Input: dimensioned drawing with shaded views. Units: mm. Origin: part minimum x, y, z. A direction names the side the tool comes from. Round coordinates to 2 decimals unless told otherwise and drop trailing zeros. Write each loop counter-clockwise with the first axis right and the second up, starting at its lowest first coordinate (ties: lowest second). Pieces come first, ordered by that corner, then holes. Notation, with made-up numbers: M -13.75,87.25 L 13.25,87.25 A33 ccw 13.25,115.25 Z; hole C 59,36 d9. An arc over 180 degrees is marked long. Answer as CSV lines item,"result". Start each with the question number.
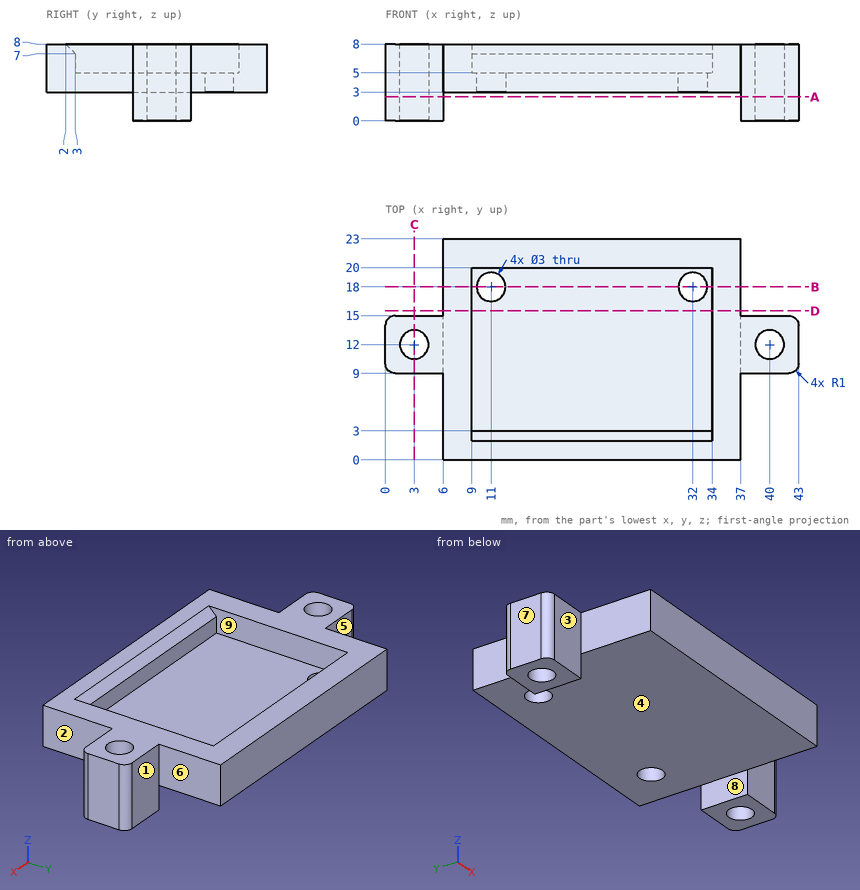
Item 1: Cut plane B-B, the plane y = 18. Return loops of the section in (x, z).
Item 2: Cut plane A-A, the plane z = 2.5. Return loops of the section in (x, y).
Item 3: Pin query (flat end, axial travel): pin 1 Ø1 at (x, y) = (24.5, 17) entering from +Z; pin 2 Ø7 at (x, y) = (15.5, 9.5) entering from -Z; pin 3 Ø2.5 at (x, z) = (38.5, 5) entering from -Y; pin 4 Ø2.5 at (x, y) = (11, 18) entering from -Z. Return the tip coordinate at first contact, or that it passes through.
Item 4: Line query: line 1 (Y direction, x = 3, z = 4.25); line 2 (Y direction, x = 17, z = 5.75); line 3 (X direction, y = 16.75, z = 3.25). Output: solid intervals per line, ascending. Write a range as [from, to].
Item 5: Cut plane D-D, the plane y = 15.5. Return loops of the section in (x, z).
Item 6: Access query for the marked faces 1, 2, 3, 4 and 5. Directions: +Z, -Z, +X, -X, +Y, -Y. A direction counts if a zero-diameter tool reaches every point of the face in a straight line with its end or side. Return the directions, or none.
Item 7: Draft query along X for the marked faces 6, 7, 8 and 9. Return one class per face: +X half, -X half, draft (parallel to the pull), parting line (faces both ways), or undercut.
Item 8: Cut plane C-C, the plane x = 3. Return loops of the section in (y, z), plus the area to 3 significant figures.
Results list:
1,outline,"M 6,3 L 9.5,3 L 9.5,5 L 9,5 L 9,8 L 6,8 Z; M 12.5,3 L 30.5,3 L 30.5,5 L 12.5,5 Z; M 33.5,3 L 37,3 L 37,8 L 34,8 L 34,5 L 33.5,5 Z"
2,outline,"M 0,10 A1 ccw 1,9 L 6,9 L 6,15 L 1,15 A1 ccw 0,14 Z; M 37,9 L 42,9 A1 ccw 43,10 L 43,14 A1 ccw 42,15 L 37,15 Z; hole C 3,12 d3; hole C 40,12 d3"
3,pin 1,"z = 5"
3,pin 2,"z = 3"
3,pin 3,"y = 9"
3,pin 4,"through"
4,line 1,"[9, 10.5], [13.5, 15]"
4,line 2,"[0, 3], [20, 23]"
4,line 3,"[6, 10.17], [11.83, 31.17], [32.83, 37]"
5,outline,"M 6,3 L 37,3 L 37,8 L 34,8 L 34,5 L 9,5 L 9,8 L 6,8 Z"
6,face 1,"+Z, -Z, +X, +Y"
6,face 2,"+Z, -Z, +X, -Y"
6,face 3,"+Z, -Z, -X, -Y"
6,face 4,"-Z, +Y, -Y"
6,face 5,"+Z, -Z, -X, +Y"
7,face 6,"+X half"
7,face 7,"-X half"
7,face 8,"undercut"
7,face 9,"undercut"
8,outline,"M 9,0 L 10.5,0 L 10.5,8 L 9,8 Z; M 13.5,0 L 15,0 L 15,8 L 13.5,8 Z"
8,area,"24.0 mm²"
